from build123d import *

# Parameters (mm, degrees)
F1_W          = 23
F1_H          = 23
F2_W          = 18
F2_H          = 18
F4_T          = -1.5
F5_W          = 7
F5_H          = 2
F6_DEPTH      = 11.5010001
F6_DEPTH_BACK = 11.5010001
F7_R          = 0.9999


# Not quite as in the source:
# - a fillet or chamfer is up to 0.001 mm smaller than in the source, because OpenCascade refuses the exact size


with BuildPart() as f3:
    # F1 (on Top) → F3 section 0
    with BuildSketch(Plane.XY):
        Rectangle(F1_W, F1_H)
    # F2 (on offset) → F3 section 1
    with BuildSketch(Plane.XY.offset(23)):
        Rectangle(F2_W, F2_H)
    loft()

    # F4
    f4_openings = [f3.faces().sort_by_distance(p)[0] for p in [
        (0, 0, 0),
    ]]
    offset(amount=F4_T, openings=f4_openings)

    # F5 (on Front) → F6 (cut, two sides)
    with BuildSketch(Plane.XZ) as f6_sk:
        with Locations((0, 19.5)):
            Rectangle(F5_W, F5_H)
    extrude(amount=-F6_DEPTH, mode=Mode.SUBTRACT)
    extrude(f6_sk.sketch, amount=F6_DEPTH_BACK, mode=Mode.SUBTRACT)

    # F7 (radius 1 in the source; OpenCascade refuses exactly that, so slightly less here)
    f7_edges = [f3.edges().sort_by_distance(p)[0] for p in [
        (-3.5, 8.517322, 20.5),
        (-3.5, -8.517322, 20.5),
        (-3.5, 8.734713, 18.5),
        (-3.5, -8.734713, 18.5),
        (3.5, 8.734713, 18.5),
        (3.5, -8.734713, 18.5),
        (3.5, 8.517322, 20.5),
        (3.5, -8.517322, 20.5),
    ]]
    fillet(f7_edges, radius=F7_R)


solid = f3.part
Input: part model. Units: mm. Frame: model coordinates. A direction names the side the tool comes from. Round coordinates to 2 decimals unless told otherwise and drop trailing zeros.
1. Material intervals for line 1 (X direction, y = 1.25, z = 19.5); line 2 (Z direction, x = 7, y = 1.75); line 3 (X direction, y = 2.5, z = 20.5), sorted ascending.
The answers:
line 1: x = -9.38 to -7.87, 7.87 to 9.38
line 2: z = 21.5 to 23
line 3: x = -9.27 to -7.76, 7.76 to 9.27
2. Pin query (flat end, axial travel): P1, Ø12, axis at y = 7.5, z = 14, coming from the -X side; P2, Ø4, axis at y = -8, z = 2.5, coming from the -X side; P3, Ø1.5, axis at x = -2, z = 4.5, coming from the -Y side. Return the tip coordinate at first contact, or that it passes through.
The answers:
P1: stops at x = -10.63
P2: stops at x = -11.45
P3: stops at y = -11.09
3. Cut plane A-A, the plane x = 0.5. State how many separate pieces and enclosed holes the cut face has, then the cut area to 3 significant figures.
The answers:
separate pieces: 3
enclosed holes: 0
area: 86.1 mm2
4. Set-up query: faces 3 (the face through (-0.1, -10.2, 0)), 4 (the face through (0, 0, 21.5)), 5 (the face through (-3.199, -8.583, 20.215)). Return all of +Z, -Z, +X, -X, +Y, -Y with unobstructed straight access to the full face (end or side cutting, diameter ignored); none if empty.
The answers:
face 3: -Z, +X, -X, +Y, -Y
face 4: -Z
face 5: +Y, -Y
5. Mould query, pull axis Y, two halves, no side actions, for faces 1 (the face through (0.14, 8.806, 10.901)), 2 (the face through (-3.199, -8.692, 18.785)). Classes: released by +Y, released by -Y, zero draft, split by the parting line, or undercut.
The answers:
face 1: undercut
face 2: zero draft
